```python
from build123d import *

# Parameters (mm, degrees)
BOSS_EXTRUDE1_DEPTH  = 20
BOSS_EXTRUDE2_DEPTH  = 50
CUT_EXTRUDE1_DEPTH   = 47
CUT_EXTRUDE2_DEPTH   = 4
LPATTERN1_COUNT      = 4
LPATTERN1_PITCH      = 10
MIRROR2_COPY_1_DEPTH = 4
MIRROR2_COPY_2_DEPTH = 4
MIRROR2_COPY_3_DEPTH = 4
CUT_EXTRUDE3_DEPTH   = 30


with BuildPart() as part:
    # Sketch1 → Boss-Extrude1 (new body)
    with BuildSketch(Plane.XY):
        with BuildLine():
            ThreePointArc((-4.288832517, 8.7042), (-2.742571539, 7.105968455), (-4.274927306, 5.4944))
            Line((-4.274927306, 5.4944), (-6.476788598, 5.4944))
            ThreePointArc((-6.476788598, 5.4944), (-6.970173245, 5.164526769), (-6.853887321, 4.582528193))
            Line((-6.853887321, 4.582528193), (-3.545123878, 1.281326675))
            ThreePointArc((-3.545123878, 1.281326675), (-2.678042762, 0.703037101), (-1.655778399, 0.5))
            Line((-1.655778399, 0.5), (0, 0.5))
            Line((0, 0.5), (0, 8.7042))
            Line((0, 8.7042), (-4.288832517, 8.7042))
        make_face()
    boss_extrude1 = extrude(amount=BOSS_EXTRUDE1_DEPTH)

    # Sketch2 → Boss-Extrude2 (add)
    with BuildSketch(Plane(origin=(0, 8.7042, 0), x_dir=(1, 0, 0), z_dir=(0, 1, 0))):
        with BuildLine():
            Line((0, -20), (-23, -20))
            ThreePointArc((-23, -20), (-24.414213562, -19.414213562), (-25, -18))
            Line((-25, -18), (-25, -2))
            ThreePointArc((-25, -2), (-24.414213562, -0.585786438), (-23, 0))
            Line((-23, 0), (0, 0))
            Line((0, 0), (0, -20))
        make_face()
    boss_extrude2 = extrude(amount=BOSS_EXTRUDE2_DEPTH)

    # Sketch4 → Cut-Extrude1 (cut)
    with BuildSketch(Plane(origin=(0, 58.7042, 0), x_dir=(1, 0, 0), z_dir=(0, 1, 0))):
        Polygon((-22, -17), (-22, -3), (-19, -4), (-19, 0), (0, 0), (0, -20), (-19, -20), (-19, -16), align=None)
    cut_extrude1 = extrude(amount=-CUT_EXTRUDE1_DEPTH, mode=Mode.SUBTRACT)

    # Sketch6 → Cut-Extrude2 (cut, through all)
    with BuildSketch(Plane(origin=(-22, 0, 0), x_dir=(0, 0, -1), z_dir=(1, 0, 0))):
        with BuildLine():
            Line((-15, 19.9542), (-5, 19.9542))
            ThreePointArc((-5, 19.9542), (-10, 14.9542), (-15, 19.9542))
        make_face()
    cut_extrude2 = extrude(amount=-CUT_EXTRUDE2_DEPTH, mode=Mode.SUBTRACT)

    # LPattern1: Cut-Extrude2 ×4
    with Locations(*[(0, i * LPATTERN1_PITCH, 0) for i in range(1, LPATTERN1_COUNT)]):
        add(cut_extrude2, mode=Mode.SUBTRACT)

    # Mirror2: Boss-Extrude1, Boss-Extrude2, Cut-Extrude1, Cut-Extrude2 across Right Plane
    add(boss_extrude1.mirror(Plane(origin=(0, 0, 0), x_dir=(0, 0, -1), z_dir=(1, 0, 0))))
    add(boss_extrude2.mirror(Plane(origin=(0, 0, 0), x_dir=(0, 0, -1), z_dir=(1, 0, 0))))
    add(cut_extrude1.mirror(Plane(origin=(0, 0, 0), x_dir=(0, 0, -1), z_dir=(1, 0, 0))), mode=Mode.SUBTRACT)
    add(cut_extrude2.mirror(Plane(origin=(0, 0, 0), x_dir=(0, 0, -1), z_dir=(1, 0, 0))), mode=Mode.SUBTRACT)

    # Mirror2 copy 1 sketch → Mirror2 copy 1 (cut, through all)
    with BuildSketch(Plane(origin=(22, 10, 0), x_dir=(0, 0, -1), z_dir=(-1, 0, 0))):
        with BuildLine():
            Line((-15, -19.9542), (-5, -19.9542))
            ThreePointArc((-5, -19.9542), (-10, -14.9542), (-15, -19.9542))
        make_face()
    extrude(amount=-MIRROR2_COPY_1_DEPTH, mode=Mode.SUBTRACT)

    # Mirror2 copy 2 sketch → Mirror2 copy 2 (cut, through all)
    with BuildSketch(Plane(origin=(22, 20, 0), x_dir=(0, 0, -1), z_dir=(-1, 0, 0))):
        with BuildLine():
            Line((-15, -19.9542), (-5, -19.9542))
            ThreePointArc((-5, -19.9542), (-10, -14.9542), (-15, -19.9542))
        make_face()
    extrude(amount=-MIRROR2_COPY_2_DEPTH, mode=Mode.SUBTRACT)

    # Mirror2 copy 3 sketch → Mirror2 copy 3 (cut, through all)
    with BuildSketch(Plane(origin=(22, 30, 0), x_dir=(0, 0, -1), z_dir=(-1, 0, 0))):
        with BuildLine():
            Line((-15, -19.9542), (-5, -19.9542))
            ThreePointArc((-5, -19.9542), (-10, -14.9542), (-15, -19.9542))
        make_face()
    extrude(amount=-MIRROR2_COPY_3_DEPTH, mode=Mode.SUBTRACT)

    # Sketch7 → Cut-Extrude3 (cut)
    with BuildSketch(Plane.XY.offset(20)):
        Polygon((-2, 3.5), (0, 5.5), (2, 3.5), (0, 2.75), align=None)
    extrude(amount=-CUT_EXTRUDE3_DEPTH, mode=Mode.SUBTRACT)


solid = part.part
```
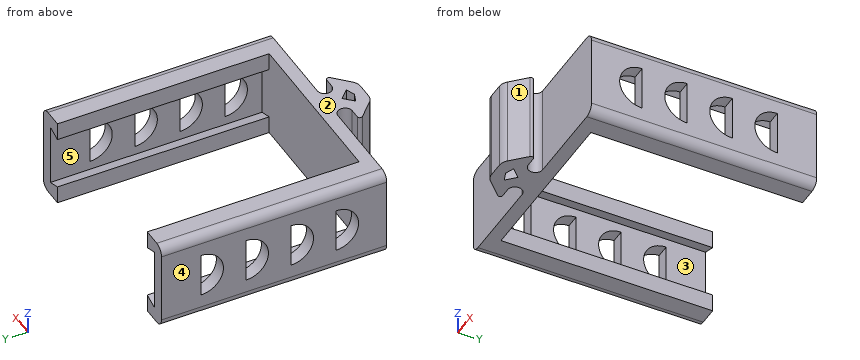
Build history of the part. All positions in model axes, mm. Face numbers are marked on the shaded views. A direction names the side the tool comes from. Round coordinates to 2 decimals unless told otherwise and drop trailing zeros. Order: outer loops, then holes, each group sorted by start corner. A loop starts at its lowest first (then second) coordinate and runs counter-clockwise, first axis right, second up. Notation, with made-up numbers: (45.5, 3.25) -> (70.5, 3.25) arc R21 cw to (70.5, 10.25) -> close; hole circle Ø1 at (7.5, 69). An arc over 180 degrees is marked (long way). Answer in a Markdown table with one row per item.
1) Band-saw the part on D-D on x = 10. Give the cut face in (y, z), and give its area (3 significant figures).
Values:
| item | result |
|---|---|
| outline | (8.7, 0) -> (11.7, 0) -> (11.7, 20) -> (8.7, 20) -> close |
| area | 60.0 mm2 |
2) Wall check: L1, parallel to X at y = 18, z = 18; L2, parallel to Y at x = 15, z = 6.25; L3, parallel to Z at x = 21.5, y = 26.5. Give the ranges that are in metal, low to high.
Values:
| item | result |
|---|---|
| L1 | -25 to -19, 19 to 25 |
| L2 | 8.7 to 11.7 |
| L3 | 0 to 3.17, 16.83 to 20 |
3) Which spindle directions (+Z, -Z, +X, -X, +Y, -Y) get a long thin tool onto all of the face, cutting with end or side? Do the marked faces 4 and 5. Say none if no direction does.
Values:
| item | result |
|---|---|
| face 4 | +Z, -Z, -X, +Y, -Y |
| face 5 | +Y |
4) Mould opens along X. For the marked faces 1, 2 and 3 say: released by +X, released by -X, zero draft, split by the parting line, or undercut.
Values:
| item | result |
|---|---|
| face 1 | released by +X |
| face 2 | zero draft |
| face 3 | undercut |
5) Band-saw the part on B-B on z = 10. Give the number of separate pieces and of enclosed holes in the cut face, and give its area (3 significant figures).
Values:
| item | result |
|---|---|
| separate pieces | 9 |
| enclosed holes | 1 |
| area | 378 mm2 |
6) Pin check, flat tips, straight feed: P1, Ø2.5, axis at x = 5.5, z = 6.5, coming from the +Y side; P2, Ø3.5, axis at x = -23.5, z = 8.5, coming from the -Y side; P3, Ø4, axis at x = -8.5, z = 17, coming from the -Y side; P4, Ø1.5, axis at x = 5.5, y = 12.5, coming from the +Z side. Stop position of each tip, or through.
Values:
| item | result |
|---|---|
| P1 | y = 11.7 |
| P2 | y = 8.7 |
| P3 | y = 4.23 |
| P4 | through |
7) Band-saw the part on A-A on y = 13. Give the cut face in (x, z), and give its area (3 significant figures).
Values:
| item | result |
|---|---|
| outline | (-25, 2) arc R2 ccw to (-23, 0) -> (-19, 0) -> (-19, 4) -> (-22, 3) -> (-22, 17) -> (-19, 16) -> (-19, 20) -> (-23, 20) arc R2 ccw to (-25, 18) -> close; (19, 0) -> (23, 0) arc R2 ccw to (25, 2) -> (25, 18) arc R2 ccw to (23, 20) -> (19, 20) -> (19, 16) -> (22, 17) -> (22, 3) -> (19, 4) -> close |
| area | 159 mm2 |
8) Band-saw the part on C-C on y = 28. Give the cut face in (x, z).
Values:
| item | result |
|---|---|
| outline | (-25, 2) arc R2 ccw to (-23, 0) -> (-19, 0) -> (-19, 4) -> (-22, 3) -> (-22, 5.4) -> (-25, 5.4) -> close; (-25, 14.6) -> (-22, 14.6) -> (-22, 17) -> (-19, 16) -> (-19, 20) -> (-23, 20) arc R2 ccw to (-25, 18) -> close; (19, 0) -> (23, 0) arc R2 ccw to (25, 2) -> (25, 5.4) -> (22, 5.4) -> (22, 3) -> (19, 4) -> close; (19, 16) -> (22, 17) -> (22, 14.6) -> (25, 14.6) -> (25, 18) arc R2 ccw to (23, 20) -> (19, 20) -> close |
